```python
from build123d import *

# Parameters (mm, degrees)
BASE_FLANGE2_DEPTH = 101.6
CUT_EXTRUDE1_DEPTH = 1.27


# Sheet-metal steps are written as plain solids
with BuildPart() as part:
    # Sketch1 → Base-Flange2 (new body)
    with BuildSketch(Plane(origin=(0, 0, 0), x_dir=(1, 0, 0), z_dir=(0, 1, 0))):
        with BuildLine():
            Line((12.954, 0), (22.1234, 0))
            ThreePointArc((22.1234, 0), (24.440306079, 0.959693921), (25.4, 3.2766))
            Line((25.4, 3.2766), (25.4, 11.9634))
            ThreePointArc((25.4, 11.9634), (24.440306079, 14.280306079), (22.1234, 15.24))
            Line((22.1234, 15.24), (3.2766, 15.24))
            ThreePointArc((3.2766, 15.24), (0.959693921, 14.280306079), (0, 11.9634))
            Line((0, 11.9634), (0, 3.2766))
            ThreePointArc((0, 3.2766), (0.959693921, 0.959693921), (3.2766, 0))
            Line((3.2766, 0), (12.446, 0))
            Line((12.446, 0), (12.446, 2.54))
            Line((12.446, 2.54), (3.2766, 2.54))
            ThreePointArc((3.2766, 2.54), (2.755745145, 2.755745145), (2.54, 3.2766))
            Line((2.54, 3.2766), (2.54, 11.9634))
            ThreePointArc((2.54, 11.9634), (2.755745145, 12.484254855), (3.2766, 12.7))
            Line((3.2766, 12.7), (22.1234, 12.7))
            ThreePointArc((22.1234, 12.7), (22.644254855, 12.484254855), (22.86, 11.9634))
            Line((22.86, 11.9634), (22.86, 3.2766))
            ThreePointArc((22.86, 3.2766), (22.644254855, 2.755745145), (22.1234, 2.54))
            Line((22.1234, 2.54), (12.954, 2.54))
            Line((12.954, 2.54), (12.954, 0))
        make_face()
    extrude(amount=BASE_FLANGE2_DEPTH)

    # Sketch2 → Cut-Extrude1 (cut)
    with BuildSketch(Plane(origin=(0, 0, -15.24), x_dir=(-1, 0, 0), z_dir=(0, 0, -1))):
        Polygon((-17.544402312, 4.806950327), (-17.259466414, 4.806950327), (-17.259466414, 3.597880815), (-15.93591373, 4.806950327), (-15.529498466, 4.806950327), (-17.089649708, 3.38227084), (-15.407383081, 1.631950327), (-15.787085605, 1.631950327), (-17.259466414, 3.164116793), (-17.259466414, 1.631950327), (-17.544402312, 1.631950327), align=None)
        Polygon((-14.939274107, 4.806950327), (-14.654338209, 4.806950327), (-14.654338209, 1.957591352), (-13.433184363, 1.957591352), (-13.433184363, 1.631950327), (-14.939274107, 1.631950327), align=None)
        Polygon((-13.107543337, 4.806950327), (-12.813067176, 4.806950327), (-12.191677953, 2.47848979), (-11.267544339, 4.806950327), (-11.226203193, 4.806950327), (-10.319242055, 2.494390231), (-9.694672744, 4.806950327), (-9.403376671, 4.806950327), (-10.259456398, 1.631950327), (-10.300161526, 1.631950327), (-11.255460004, 4.060265631), (-12.222206799, 1.631950327), (-12.262911927, 1.631950327), align=None)
        Polygon((-8.996325389, 4.481309301), (-8.996325389, 4.806950327), (-7.327415132, 4.806950327), (-8.659236046, 1.957591352), (-7.36812026, 1.957591352), (-7.36812026, 1.631950327), (-9.118440773, 1.631950327), (-7.78661986, 4.481309301), align=None)
    extrude(amount=-CUT_EXTRUDE1_DEPTH, mode=Mode.SUBTRACT)


solid = part.part
```
Design review of the part built by this model. Coordinates are the model's own, in mm. A direction names the side the tool comes from. Give positions to 0.01 mm unless a question says otherwise; leave off trailing zeros. Loops run counter-clockwise (first coordinate to the right, second up) from the corner with the lowest first, then second, coordinate; pieces in that order, holes last. Notation, with made-up numbers: (68, 60) -> (115, 60) arc R14 ccw to (115, 64) -> close; hole circle Ø2 at (-30, 31.25). An arc over 180 degrees is marked (long way). One line per item, written item: value.
Q1. For L1, parallel to X at y = 88, z = -11; L2, parallel to Z at x = 15.5, y = 38; L3, parallel to X at y = 18.5, z = -1.75, list the stretches that pass through material, from the lowest coordinate up.
Numbers:
L1: x = 0 to 2.54, 22.86 to 25.4
L2: z = -15.24 to -12.7, -2.54 to 0
L3: x = 0.38 to 12.45, 12.95 to 25.02
Q2. For pin 1 Ø1 at (y, z) = (2.5, -14.5) entering from +X; pin 2 Ø2 at (y, z) = (53, -1) entering from +X; pin 3 Ø1.3 at (y, z) = (57, -1) entering from -X, all flat-tipped, find the tip position at first contact; note any pin that passes through.
Numbers:
pin 1: stops at x = 24.69
pin 2: stops at x = 25.14
pin 3: stops at x = 0.43
Q3. We need section B-B on x = 20.75. Give the boundary of the cut face in (y, z), and give its area (3 significant figures).
Numbers:
outline: (0, -15.24) -> (101.6, -15.24) -> (101.6, -12.7) -> (0, -12.7) -> close; (0, -2.54) -> (101.6, -2.54) -> (101.6, 0) -> (0, 0) -> close
area: 516 mm^2
Q4. Machinability: for faces 1 (the flat face through (2.54, 50, -8)), 2 (the flat face through (25.4, 50, -8)), 3 (the flat face through (12.446, 50, -1)), which of the approach directions +Z, -Z, +X, -X, +Y, -Y give a long, thin tool a straight path to every point of the face, cutting with its end or side? Answer none if there is none.
Numbers:
face 1: +Y, -Y
face 2: +Z, -Z, +X, +Y, -Y
face 3: +Z, +Y, -Y
Q5. We need section A-A on z = -9.75. Give the boundary of the cut face in (x, y), and give its area (3 significant figures).
Numbers:
outline: (0, 0) -> (2.54, 0) -> (2.54, 101.6) -> (0, 101.6) -> close; (22.86, 0) -> (25.4, 0) -> (25.4, 101.6) -> (22.86, 101.6) -> close
area: 516 mm^2
Q6. We need section C-C on y = 92.5. Give the boundary of the cut face in (x, z), and give its area (3 significant figures).
Numbers:
outline: (0, -11.96) arc R3.28 ccw to (3.28, -15.24) -> (22.12, -15.24) arc R3.28 ccw to (25.4, -11.96) -> (25.4, -3.28) arc R3.28 ccw to (22.12, 0) -> (12.95, 0) -> (12.95, -2.54) -> (22.12, -2.54) arc R0.74 cw to (22.86, -3.28) -> (22.86, -11.96) arc R0.74 cw to (22.12, -12.7) -> (3.28, -12.7) arc R0.74 cw to (2.54, -11.96) -> (2.54, -3.28) arc R0.74 cw to (3.28, -2.54) -> (12.45, -2.54) -> (12.45, 0) -> (3.28, 0) arc R3.28 ccw to (0, -3.28) -> close
area: 171 mm^2
Q7. Draft analysis for pull direction Z (two halves, no side actions). For faces 4 (the flat face through (12.954, 50, -1)), 5 (the flat face through (22.86, 50, -8)), 6 (the cylindrical face through (24.47, 50.09, -14.25)), 7 (the flat face through (18, 50, -2.54)), state which applies: pulls with the +Z half, pulls with the -Z half, needs draft (parallel to the pull), parting line crosses it, or undercut.
Numbers:
face 4: needs draft
face 5: undercut
face 6: pulls with the -Z half
face 7: undercut
